Could you check a few things on this model? Use its own coordinates, in mm. Coordinates: 2 decimals unless noted, no trailing zeros. Order: outer loops, then holes, each group sorted by start corner. A loop starts at its lowest first (then second) coordinate and runs counter-clockwise, first axis right, second up. Notation, with made-up numbers: (8, -36) -> (30, -36) arc R17 cw to (30, -7) -> close; hole circle Ø8 at (43, -10.75). An arc over 180 degrees is marked (long way). Use a Markdown table: item, result. Add a question column.
1) If we section it at A-A (x = 289): Write out the boundary of the cut face in (y, z), plus the area to 3 significant figures.
2) If we section it at B-B (y = 28): Write out the boundary of the cut face in (x, z).
3) If we section it at C-C (y = 62): Write out the boundary of the cut face in (x, z).
4) Will these pins go through, and if not, where does the flat tip stop? pin 1 Ø2 at (y, z) = (2, -6) entering from -X; pin 2 Ø0.6 at (x, y) = (254.5, 2) entering from -Z.
5) If I drill on L1, parallel to Z at x = 260, y = 2; L2, parallel to X at y = 139, z = -7; L3, parallel to Z at x = 0.7, y = 28, over which ranges is the centre line in solid material (lowest first)? Write a range as [from, to].
```python
from build123d import *

# Parameters (mm, degrees)
EXTRUDE022_DEPTH        = 11
SKETCH124_W             = 3
SKETCH124_H             = 12.5
SKETCH124_H_2           = 3
EXTRUDE114_DEPTH        = 6
SKETCH126_R             = 1.28
EXTRUDE116_DEPTH        = 10
BODY064_PLACEMENT_ANGLE = 90
BODY068_PLACEMENT_ANGLE = 90
BODY069_PLACEMENT_ANGLE = 90
BODY070_PLACEMENT_ANGLE = 90
BODY071_PLACEMENT_ANGLE = 90
BODY072_ROLL_ANGLE      = -90
BODY072_PLACEMENT_ANGLE = 90
BODY076_ROLL_ANGLE      = -90
BODY076_PLACEMENT_ANGLE = -90
BODY077_ROLL_ANGLE      = -90
BODY077_PLACEMENT_ANGLE = 90
BODY078_ROLL_ANGLE      = -90
BODY078_PLACEMENT_ANGLE = 180
BODY079_ROLL_ANGLE      = -90
BODY079_PLACEMENT_ANGLE = 180
BODY086_PLACEMENT_ANGLE = 90
BODY087_PLACEMENT_ANGLE = 90
BODY088_PLACEMENT_ANGLE = 90
BODY089_PLACEMENT_ANGLE = 90
SKETCH133_R             = 6.25
EXTRUDE123_DEPTH        = 1
EXTRUDE123_DEPTH_BACK   = 10
SKETCH055_W             = 80
SKETCH055_H             = 14
SKETCH055_W_2           = 77
SKETCH055_H_2           = 11
SKETCH055_W_3           = 10
SKETCH055_H_3           = 17
EXTRUDE045_DEPTH        = 8


with BuildPart() as rear_holes002:
    # Sketch028 → Extrude022 (new body)
    with BuildSketch(Plane(origin=(0, 203, 0), x_dir=(-1, 0, 0), z_dir=(0, 1, 0))):
        Polygon((-2, -26), (-356, -26), (-356, -12), (-321.5, -12), (-321.5, -6.68), (-219, -6.68), (-219, -2), (-180.5, -2), (-180.5, -12), (-2, -12), align=None)
    extrude(amount=EXTRUDE022_DEPTH)


with BuildPart() as extrude114:
    # Sketch124 → Extrude114 (new body)
    with BuildSketch(Plane(origin=(0, 0, -26), x_dir=(1, 0, 0), z_dir=(0, 0, -1))):
        with Locations((1, -100.25)):
            Rectangle(SKETCH124_W, SKETCH124_H)
        with Locations((357, -100.25)):
            Rectangle(SKETCH124_W, SKETCH124_H)
        with Locations((126, -2)):
            Rectangle(SKETCH124_W, SKETCH124_H_2)
        with Locations((255, -2)):
            Rectangle(SKETCH124_W, SKETCH124_H_2)
    extrude(amount=-EXTRUDE114_DEPTH)


with BuildPart() as screw_inner:
    # Sketch126 → Extrude116 (new body)
    with BuildSketch(Plane.XY):
        Circle(SKETCH126_R)
    extrude(amount=EXTRUDE116_DEPTH)


with BuildPart() as screw_inner001:
    # Body064 base: copy of screw inner
    add(screw_inner.part)


with BuildPart() as screw_inner001_1:
    # Body064 placement: moved
    add(screw_inner001.part.moved(Location((-1.5, 51, -3.68))).rotate(Axis((-1.5, 51, -3.68), (0, 1, 0)), BODY064_PLACEMENT_ANGLE))


with BuildPart() as screw_inner002:
    # Body068 base: copy of screw inner
    add(screw_inner.part)


with BuildPart() as screw_inner002_1:
    # Body068 placement: moved
    add(screw_inner002.part.moved(Location((7, -1, -8.5))).rotate(Axis((7, -1, -8.5), (-1, 0, 0)), BODY068_PLACEMENT_ANGLE))


with BuildPart() as screw_inner003:
    # Body069 base: copy of screw inner
    add(screw_inner.part)


with BuildPart() as screw_inner003_1:
    # Body069 placement: moved
    add(screw_inner003.part.moved(Location((99.5, -1, -8.5))).rotate(Axis((99.5, -1, -8.5), (-1, 0, 0)), BODY069_PLACEMENT_ANGLE))


with BuildPart() as screw_inner004:
    # Body070 base: copy of screw inner
    add(screw_inner.part)


with BuildPart() as screw_inner004_1:
    # Body070 placement: moved
    add(screw_inner004.part.moved(Location((133, -1, -3.68))).rotate(Axis((133, -1, -3.68), (-1, 0, 0)), BODY070_PLACEMENT_ANGLE))


with BuildPart() as screw_inner005:
    # Body071 base: copy of screw inner
    add(screw_inner.part)


with BuildPart() as screw_inner005_1:
    # Body071 placement: moved
    add(screw_inner005.part.moved(Location((260, -1, -3.68))).rotate(Axis((260, -1, -3.68), (-1, 0, 0)), BODY071_PLACEMENT_ANGLE))


with BuildPart() as screw_inner006:
    # Body072 base: copy of screw inner
    add(screw_inner.part)


with BuildPart() as screw_inner006_1:
    # Body072 roll: moved
    add(screw_inner006.part.rotate(Axis((0, 0, 0), (1, 0, 0)), BODY072_ROLL_ANGLE))


with BuildPart() as screw_inner006_2:
    # Body072 placement: moved
    add(screw_inner006_1.part.moved(Location((360, 51, -3.68))).rotate(Axis((360, 51, -3.68), (0, 0, 1)), BODY072_PLACEMENT_ANGLE))


with BuildPart() as screw_inner007:
    # Body076 base: copy of screw inner
    add(screw_inner.part)


with BuildPart() as screw_inner007_1:
    # Body076 roll: moved
    add(screw_inner007.part.rotate(Axis((0, 0, 0), (1, 0, 0)), BODY076_ROLL_ANGLE))


with BuildPart() as screw_inner007_2:
    # Body076 placement: moved
    add(screw_inner007_1.part.moved(Location((-2, 146, -3.68))).rotate(Axis((-2, 146, -3.68), (0, 0, 1)), BODY076_PLACEMENT_ANGLE))


with BuildPart() as screw_inner008:
    # Body077 base: copy of screw inner
    add(screw_inner.part)


with BuildPart() as screw_inner008_1:
    # Body077 roll: moved
    add(screw_inner008.part.rotate(Axis((0, 0, 0), (1, 0, 0)), BODY077_ROLL_ANGLE))


with BuildPart() as screw_inner008_2:
    # Body077 placement: moved
    add(screw_inner008_1.part.moved(Location((360, 146, -3.68))).rotate(Axis((360, 146, -3.68), (0, 0, 1)), BODY077_PLACEMENT_ANGLE))


with BuildPart() as screw_inner009:
    # Body078 base: copy of screw inner
    add(screw_inner.part)


with BuildPart() as screw_inner009_1:
    # Body078 roll: moved
    add(screw_inner009.part.rotate(Axis((0, 0, 0), (1, 0, 0)), BODY078_ROLL_ANGLE))


with BuildPart() as screw_inner009_2:
    # Body078 placement: moved
    add(screw_inner009_1.part.moved(Location((134, 213, -3.68))).rotate(Axis((134, 213, -3.68), (0, 0, 1)), BODY078_PLACEMENT_ANGLE))


with BuildPart() as screw_inner010:
    # Body079 base: copy of screw inner
    add(screw_inner.part)


with BuildPart() as screw_inner010_1:
    # Body079 roll: moved
    add(screw_inner010.part.rotate(Axis((0, 0, 0), (1, 0, 0)), BODY079_ROLL_ANGLE))


with BuildPart() as screw_inner010_2:
    # Body079 placement: moved
    add(screw_inner010_1.part.moved(Location((330, 213, -3.68))).rotate(Axis((330, 213, -3.68), (0, 0, 1)), BODY079_PLACEMENT_ANGLE))


with BuildPart() as screw_inner011:
    # Body086 base: copy of screw inner
    add(screw_inner.part)


with BuildPart() as screw_inner011_1:
    # Body086 placement: moved
    add(screw_inner011.part.moved(Location((-1, 88, -21))).rotate(Axis((-1, 88, -21), (0, 1, 0)), BODY086_PLACEMENT_ANGLE))


with BuildPart() as screw_inner012:
    # Body087 base: copy of screw inner
    add(screw_inner.part)


with BuildPart() as screw_inner012_1:
    # Body087 placement: moved
    add(screw_inner012.part.moved(Location((359, 88, -21))).rotate(Axis((359, 88, -21), (0, -1, 0)), BODY087_PLACEMENT_ANGLE))


with BuildPart() as screw_inner013:
    # Body088 base: copy of screw inner
    add(screw_inner.part)


with BuildPart() as screw_inner013_1:
    # Body088 placement: moved
    add(screw_inner013.part.moved(Location((133, 0, -21))).rotate(Axis((133, 0, -21), (-1, 0, 0)), BODY088_PLACEMENT_ANGLE))


with BuildPart() as screw_inner014:
    # Body089 base: copy of screw inner
    add(screw_inner.part)


with BuildPart() as screw_inner014_1:
    # Body089 placement: moved
    add(screw_inner014.part.moved(Location((260, 0, -21))).rotate(Axis((260, 0, -21), (-1, 0, 0)), BODY089_PLACEMENT_ANGLE))


with BuildPart() as power_hole002:
    # Sketch133 → Extrude123 (new body, two sides)
    with BuildSketch(Plane(origin=(-3, 0, 0), x_dir=(0, -1, 0), z_dir=(-1, 0, 0))) as extrude123_sk:
        with Locations((-28, -10)):
            Circle(SKETCH133_R)
    extrude(amount=EXTRUDE123_DEPTH)
    extrude(extrude123_sk.sketch, amount=-EXTRUDE123_DEPTH_BACK)


with BuildPart() as compound012:
    # Sketch055 → Extrude045 (new body)
    with BuildSketch(Plane.XZ.offset(3)):
        with Locations((212, -9)):
            Rectangle(SKETCH055_W, SKETCH055_H)
        with Locations((307, -7.5)):
            Rectangle(SKETCH055_W_2, SKETCH055_H_2)
        with Locations((117, -10.5)):
            Rectangle(SKETCH055_W_3, SKETCH055_H_3)
    extrude(amount=-EXTRUDE045_DEPTH)

    # Compound012: union rear holes002, Extrude114, screw inner001, screw inner002, screw inner003, screw inner004, screw inner005, screw inner006, screw inner007, screw inner008, screw inner009, screw inner010, screw inner011, screw inner012, screw inner013, screw inner014, power hole002
    add(rear_holes002.part)
    add(extrude114.part)
    add(screw_inner001_1.part)
    add(screw_inner002_1.part)
    add(screw_inner003_1.part)
    add(screw_inner004_1.part)
    add(screw_inner005_1.part)
    add(screw_inner006_2.part)
    add(screw_inner007_2.part)
    add(screw_inner008_2.part)
    add(screw_inner009_2.part)
    add(screw_inner010_2.part)
    add(screw_inner011_1.part)
    add(screw_inner012_1.part)
    add(screw_inner013_1.part)
    add(screw_inner014_1.part)
    add(power_hole002.part)


with BuildPart() as side003:
    # Sweep001: sweep along a path in Sketch004
    with BuildLine(Plane.XY) as sweep001_path:
        Line((-0.5, 211.5), (358.5, 211.5))
        Line((358.5, 211.5), (358.5, 0.5))
        Line((358.5, 0.5), (-0.5, 0.5))
        Line((-0.5, 0.5), (-0.5, 211.5))
    # Sketch003 → Sweep001 (sweep)
    with BuildSketch(Plane.XZ.offset(-14)):
        Polygon((7, -2), (7, 0), (0, 0), (0, -24.5), (2, -24.5), (2, -2), align=None)
    sweep(path=sweep001_path.line, transition=Transition.RIGHT)

    # Cut004: cut Compound012
    add(compound012.part, mode=Mode.SUBTRACT)


solid = side003.part
```
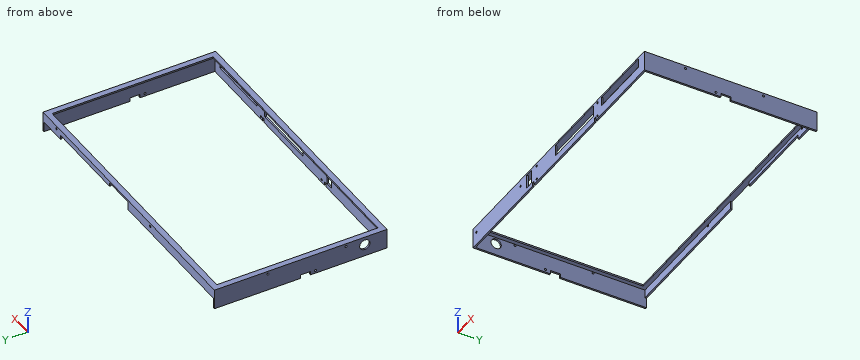
Answer sheet:
| question | item | result |
|---|---|---|
| 1 | outline | (1, -24.5) -> (3, -24.5) -> (3, -13) -> (1, -13) -> close; (1, -2) -> (8, -2) -> (8, 0) -> (1, 0) -> close; (204, -2) -> (209, -2) -> (209, -6.68) -> (211, -6.68) -> (211, 0) -> (204, 0) -> close |
| 1 | area | 60.4 mm2 |
| 2 | outline | (0, -24.5) -> (2, -24.5) -> (2, -16.25) -> (0, -16.25) -> close; (0, -3.75) -> (2, -3.75) -> (2, -2) -> (7, -2) -> (7, 0) -> (0, 0) -> close; (351, -2) -> (356, -2) -> (356, -24.5) -> (358, -24.5) -> (358, 0) -> (351, 0) -> close |
| 3 | outline | (0, -24.5) -> (2, -24.5) -> (2, -2) -> (7, -2) -> (7, 0) -> (0, 0) -> close; (351, -2) -> (356, -2) -> (356, -24.5) -> (358, -24.5) -> (358, 0) -> (351, 0) -> close |
| 4 | pin 1 | x = 0 |
| 4 | pin 2 | z = -20 |
| 5 | L1 | [-24.5, -22.28], [-19.72, -4.96], [-2.4, 0] |
| 5 | L2 | [0, 2], [356, 358] |
| 5 | L3 | [-24.5, -16.25], [-3.75, 0] |
